Input: part model. Units: mm. Frame: model coordinates. Face numbers are marked on the shaded views. A direction names the side the tool comes from. Coordinates: 2 decimals unless noted, no trailing zeros. Loops run counter-clockwise (first coordinate to the right, second up) from the corner with the lowest first, then second, coordinate; pieces in that order, holes last.
Item 1: Section A-A on z = 19.05. Return loops of the section in (x, y) (3 decimals).
Item 2: Section D-D on z = 2. Return loops of the section in (x, y).
Item 3: Contact query for flat-ended pins moving along their axis: P1, Ø1.9, axis at y = -18, z = -3.5, coming from the +X side; P2, Ø4.5, axis at x = 11, y = 5.5, coming from the -Z side (3 decimals); P3, Ø5.5, axis at x = 0, z = 19.05, coming from the -Y side; P4, Ø1, axis at x = 5, y = 8, coming from the +Z side (3 decimals). Output: stop coordinate, or through.
Item 4: Section B-B on x = 0. Return loops of the section in (y, z) (3 decimals).
Item 5: Reachability of the marked faces 4, 5, 6, 7 and 8 from +Z, -Z, +X, -X, +Y, -Y: full face, straight path, thin tool, end or side. Return the list, or none.
Item 6: Pull-direction query (Z, two-part tool) for the marked faces 1, 2 and 3; classes: released by +Z, released by -Z, zero draft, split by the parting line, or undercut.
Item 7: Section C-C on y = -12. Return loops of the section in (x, z) (1 decimal), and give its area (3 significant figures).
Item 8: Ray query, line 1 along Y through (x, z) = (-0.45, 6.35); line 2 along Z through (x, y) = (0, -19.5) (3 decimals); line 3 along Z through (x, y) = (2.5, -16). Return the intervals inside material, ascending.
```python
from build123d import *

# Parameters (mm, degrees)
SKETCH1_W            = 2.984999904
SKETCH1_H            = 41.686759908
BOSS_EXTRUDE1_DEPTH  = 12.7
SKETCH5_R            = 2
CUT_EXTRUDE2_DEPTH   = 3.984999904
SKETCH8_W            = 12.7
SKETCH8_H            = 6.35
BOSS_EXTRUDE2_DEPTH  = 12.7
SKETCH9_R            = 3.175
CUT_EXTRUDE3_DEPTH   = 12.7
SKETCH11_W           = 12.7
SKETCH11_H           = 6.35
BOSS_EXTRUDE3_DEPTH  = 12.7
CUT_EXTRUDE4_REACH   = 9.842
SKETCH12_R           = 2
SKETCH15_R           = 3
SKETCH15_R_2         = 2
BOSS_EXTRUDE5_DEPTH  = 1.5
SKETCH16_R           = 3
SKETCH16_R_2         = 2
BOSS_EXTRUDE6_DEPTH  = 1.5
SKETCH13_W           = 6.35
SKETCH13_H           = 41.686759908
SKETCH13_W_2         = 7
SKETCH13_H_2         = 6.35
BOSS_EXTRUDE4_DEPTH  = 6.35
SKETCH17_R           = 2
CUT_EXTRUDE5_DEPTH   = 29.685
SKETCH18_R           = 3
SKETCH18_R_2         = 2
BOSS_EXTRUDE7_DEPTH  = 1.5
SKETCH19_R           = 3
SKETCH19_R_2         = 2
BOSS_EXTRUDE8_DEPTH  = 1.5
CUT_EXTRUDE6_REACH   = 27.4
SKETCH20_W           = 6.35
SKETCH20_H           = 18.98776
SKETCH21_R           = 2
BOSS_EXTRUDE9_DEPTH  = 6.35
BOSS_EXTRUDE10_DEPTH = 3.175
BOSS_EXTRUDE11_DEPTH = 3.175
SKETCH24_R           = 4
CUT_EXTRUDE8_DEPTH   = 6.35
FILLET3_R            = 2


with BuildPart() as part:
    # Sketch1 → Boss-Extrude1 (new body)
    with BuildSketch(Plane.XY):
        Rectangle(SKETCH1_W, SKETCH1_H)
    extrude(amount=BOSS_EXTRUDE1_DEPTH)

    # Sketch5 → Cut-Extrude2 (cut, through all)
    with BuildSketch(Plane(origin=(1.492499952, 0, 0), x_dir=(0, 0, -1), z_dir=(1, 0, 0))):
        with Locations((-6.35, 14.493379954)):
            Circle(SKETCH5_R)
    extrude(amount=-CUT_EXTRUDE2_DEPTH, mode=Mode.SUBTRACT)

    # Sketch8 → Boss-Extrude2 (add)
    with BuildSketch(Plane.XY.offset(12.7)):
        with Locations((0, -17.668379954)):
            Rectangle(SKETCH8_W, SKETCH8_H)
    boss_extrude2 = extrude(amount=BOSS_EXTRUDE2_DEPTH)

    # Sketch9 → Cut-Extrude3 (cut)
    with BuildSketch(Plane(origin=(0, -14.493379954, 0), x_dir=(1, 0, 0), z_dir=(0, 1, 0))):
        with Locations((0, -19.05)):
            Circle(SKETCH9_R)
    cut_extrude3 = extrude(amount=-CUT_EXTRUDE3_DEPTH, mode=Mode.SUBTRACT)

    # Mirror1: Boss-Extrude2, Cut-Extrude3 across plane
    add(boss_extrude2.mirror(Plane(origin=(0, 0, 6.35), x_dir=(1, 0, 0), z_dir=(0, 0, -1))))
    add(cut_extrude3.mirror(Plane(origin=(0, 0, 6.35), x_dir=(1, 0, 0), z_dir=(0, 0, -1))), mode=Mode.SUBTRACT)

    # Sketch11 → Boss-Extrude3 (add)
    with BuildSketch(Plane(origin=(0, 0, 12.7), x_dir=(-1, 0, 0), z_dir=(0, 0, -1))):
        with Locations((0, -17.668379954)):
            Rectangle(SKETCH11_W, SKETCH11_H)
    extrude(amount=BOSS_EXTRUDE3_DEPTH)

    # Sketch12 → Cut-Extrude4 (cut, up to next)
    with BuildSketch(Plane(origin=(1.492499952, 0, 0), x_dir=(0, 0, -1), z_dir=(1, 0, 0)), mode=Mode.PRIVATE) as cut_extrude4_sk1:
        with Locations((-6.35, -3.144380046)):
            Circle(SKETCH12_R)
    cut_extrude4_tool1 = extrude(cut_extrude4_sk1.sketch, amount=-CUT_EXTRUDE4_REACH, mode=Mode.PRIVATE) & part.part
    add(cut_extrude4_tool1.solids().sort_by_distance((1.4925, -3.14438, 6.35))[0], mode=Mode.SUBTRACT)

    # Sketch15 → Boss-Extrude5 (add)
    with BuildSketch(Plane.ZY.offset(1.492499952)):
        with Locations((6.35, 14.493379954)):
            Circle(SKETCH15_R)
        with Locations((6.35, 14.493379954)):
            Circle(SKETCH15_R_2, mode=Mode.SUBTRACT)
    extrude(amount=BOSS_EXTRUDE5_DEPTH)

    # Sketch16 → Boss-Extrude6 (add)
    with BuildSketch(Plane(origin=(1.492499952, 0, 0), x_dir=(0, 0, -1), z_dir=(1, 0, 0))):
        with Locations((-6.35, -3.144380046)):
            Circle(SKETCH16_R)
        with Locations((-6.35, -3.144380046)):
            Circle(SKETCH16_R_2, mode=Mode.SUBTRACT)
    extrude(amount=BOSS_EXTRUDE6_DEPTH)

    # Sketch13 → Boss-Extrude4 (add, symmetric)
    with BuildSketch(Plane(origin=(0, 0, 6.35), x_dir=(-1, 0, 0), z_dir=(0, 0, -1))):
        with Locations((-11.667499952, 0)):
            Rectangle(SKETCH13_W, SKETCH13_H)
        with Locations((-4.992499952, -17.668379954)):
            Rectangle(SKETCH13_W_2, SKETCH13_H_2)
        with Locations((11.667499952, 0)):
            Rectangle(SKETCH13_W, SKETCH13_H)
        with Locations((4.992499952, -17.668379954)):
            Rectangle(SKETCH13_W_2, SKETCH13_H_2)
    extrude(amount=BOSS_EXTRUDE4_DEPTH, both=True)

    # Sketch17 → Cut-Extrude5 (cut)
    with BuildSketch(Plane.ZY.offset(14.842499952)):
        with Locations((6.35, 14.493379954)):
            Circle(SKETCH17_R)
        with Locations((6.35, -3.144380046)):
            Circle(SKETCH17_R)
    extrude(amount=-CUT_EXTRUDE5_DEPTH, mode=Mode.SUBTRACT)

    # Sketch18 → Boss-Extrude7 (add)
    with BuildSketch(Plane.ZY.offset(-8.492499952)):
        with Locations((6.35, -3.144380046)):
            Circle(SKETCH18_R)
        with Locations((6.35, -3.144380046)):
            Circle(SKETCH18_R_2, mode=Mode.SUBTRACT)
    extrude(amount=BOSS_EXTRUDE7_DEPTH)

    # Sketch19 → Boss-Extrude8 (add)
    with BuildSketch(Plane(origin=(-8.492499952, 0, 0), x_dir=(0, 0, -1), z_dir=(1, 0, 0))):
        with Locations((-6.35, 14.493379954)):
            Circle(SKETCH19_R)
        with Locations((-6.35, 14.493379954)):
            Circle(SKETCH19_R_2, mode=Mode.SUBTRACT)
    extrude(amount=BOSS_EXTRUDE8_DEPTH)

    # Sketch20 → Cut-Extrude6 (cut, up to next)
    with BuildSketch(Plane(origin=(0, 0, 0), x_dir=(-1, 0, 0), z_dir=(0, 0, -1)), mode=Mode.PRIVATE) as cut_extrude6_sk1:
        with Locations((-11.667499952, 11.349499954)):
            Rectangle(SKETCH20_W, SKETCH20_H)
    cut_extrude6_tool1 = extrude(cut_extrude6_sk1.sketch, amount=-CUT_EXTRUDE6_REACH, mode=Mode.PRIVATE) & part.part
    add(cut_extrude6_tool1.solids().sort_by_distance((11.6675, 11.3495, 0))[0], mode=Mode.SUBTRACT)

    # Sketch21 → Boss-Extrude9 (add)
    with BuildSketch(Plane.ZY.offset(14.842499952)):
        with Locations((6.35, -3.144380046)):
            Circle(SKETCH21_R)
    extrude(amount=-BOSS_EXTRUDE9_DEPTH)

    # Sketch22 → Boss-Extrude10 (add, symmetric)
    with BuildSketch(Plane.XY.offset(6.35)):
        Polygon((8.492499952, 1.855619954), (14.842499952, 1.855619954), (14.842499952, 4.855619954), (1.492499952, 11.162706568), (1.492499952, 8.162706568), (8.492499952, 4.855619954), align=None)
    extrude(amount=BOSS_EXTRUDE10_DEPTH, both=True)

    # Sketch23 → Boss-Extrude11 (add, symmetric)
    with BuildSketch(Plane(origin=(0, 0, 6.35), x_dir=(-1, 0, 0), z_dir=(0, 0, -1))):
        Polygon((1.492499952, -7.493379954), (8.492499952, -14.493379954), (1.492499952, -14.493379954), align=None)
    extrude(amount=BOSS_EXTRUDE11_DEPTH, both=True)

    # Sketch24 → Cut-Extrude8 (cut)
    with BuildSketch(Plane(origin=(1.492499952, 0, 0), x_dir=(0, 0, -1), z_dir=(1, 0, 0))):
        with Locations((-6.35, 14.493379954)):
            Circle(SKETCH24_R)
    extrude(amount=CUT_EXTRUDE8_DEPTH, mode=Mode.SUBTRACT)

    # Fillet3
    fillet3_edges = [part.edges().sort_by_distance(p)[0] for p in [
        (14.842499952, 4.855619954, 6.35),
    ]]
    fillet(fillet3_edges, radius=FILLET3_R)


solid = part.part
```
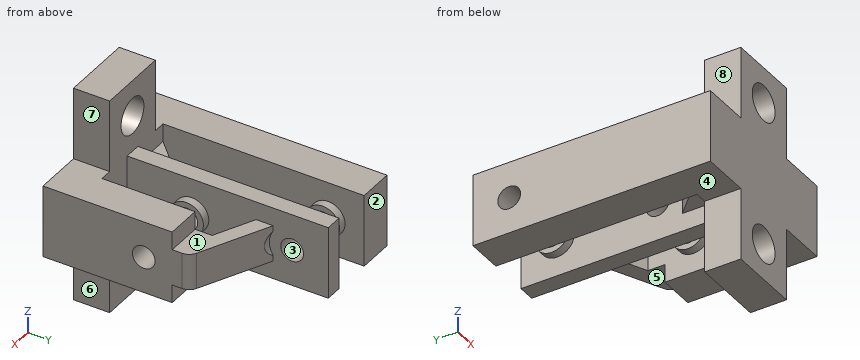
Results found:
1. outline: (-6.35, -20.843) - (-3.175, -20.843) - (-3.175, -14.493) - (-6.35, -14.493) - close; (3.175, -20.843) - (6.35, -20.843) - (6.35, -14.493) - (3.175, -14.493) - close
2. outline: (-14.84, -20.84) - (14.84, -20.84) - (14.84, 1.86) - (8.49, 1.86) - (8.49, -14.49) - (1.49, -14.49) - (1.49, 20.84) - (-1.49, 20.84) - (-1.49, -14.49) - (-8.49, -14.49) - (-8.49, 20.84) - (-14.84, 20.84) - close
3. P1: stops at x = 6.35
3. P2: stops at z = 3.175
3. P3: passes through
3. P4: stops at z = 9.525
4. outline: (-20.843, -12.7) - (-14.493, -12.7) - (-14.493, -9.525) - (-20.843, -9.525) - close; (-20.843, -3.175) - (-14.493, -3.175) - (-14.493, 0) - (20.843, 0) - (20.843, 12.7) - (-14.493, 12.7) - (-14.493, 15.875) - (-20.843, 15.875) - close; (-20.843, 22.225) - (-14.493, 22.225) - (-14.493, 25.4) - (-20.843, 25.4) - close; hole circle Ø4 at (-3.144, 6.35); hole circle Ø4 at (14.493, 6.35)
5. face 4: -Z, -X, +Y, -Y
5. face 5: -Z, +X, +Y
5. face 6: -Z, +X, +Y, -Y
5. face 7: +Z, +X, +Y, -Y
5. face 8: +Z, -X, +Y, -Y
6. face 1: released by +Z
6. face 2: zero draft
6. face 3: undercut
7. outline: (-14.8, 0) - (-8.5, 0) - (-8.5, 12.7) - (-14.8, 12.7) - close; (-6, 3.2) - (-1.5, 3.2) - (-1.5, 0) - (1.5, 0) - (1.5, 12.7) - (-1.5, 12.7) - (-1.5, 9.5) - (-6, 9.5) - close; (8.5, 0) - (14.8, 0) - (14.8, 12.7) - (8.5, 12.7) - close
7. area: 228 mm2
8. line 1: y = -20.84 to -5.14, -1.14 to 12.49, 16.49 to 20.84
8. line 2: z = -12.7 to -9.525, -3.175 to 15.875, 22.225 to 25.4
8. line 3: z = -12.7 to -8.31, -4.39 to 17.09, 21.01 to 25.4
